Geometry: final body of the model. Coordinates: model frame, mm. Face numbers are marked on the shaded views. A direction names the side the tool comes from. Give positions to 0.01 mm unless a question says otherwise; leave off trailing zeros. Write each loop counter-clockwise with the first axis right and the second up, starting at its lowest first coordinate (ties: lowest second). Pieces come first, ordered by that corner, then holes.
Q1. Cut plane B-B on x = 18.5. Return the cut outline in (y, z).
Q2. Cut plane D-D on x = 40. Return the cut outline in (y, z), plus the area to 3 significant figures.
Q3. Line query: L1, parallel to Y at x = 27, z = 12.5; L2, parallel to Z at x = 16, y = 11; L3, parallel to X at y = 2.5, z = 21.5. Output: solid intervals per line, ascending.
Q4. Reachability of the marked faces 4, 5 and 6 from +Z, -Z, +X, -X, +Y, -Y: full face, straight path, thin tool, end or side. Return the list, or none.
Q5. Draft query along X for the marked faces 1, 2 and 3. Return one class per face: pulls with the +X half, pulls with the -X half, needs draft (parallel to the pull), parting line crosses it, or undercut.
Q6. Cut plane A-A on z = 10.5. Return the cut outline in (x, y), plus the area to 3 significant figures.
Q7. Pin query (flat end, axial travel): pin 1 (5 mm diameter, centred on y = 5, z = 16, fed in from -X); pin 2 (1.5 mm diameter, centred on x = 18, z = 11, fed in from -Y); pin 3 (16 mm diameter, centred on x = 15, z = 11.5, fed in from +Y); pin 4 (6 mm diameter, centred on y = 13, z = 7.5, fed in from +X). Return the tip coordinate at first contact, or that it passes through.
```python
from build123d import *

# Parameters (mm, degrees)
F1_DEPTH  = 32
F2_R      = 16
F3_R      = 15.99999
F4_R      = 16
F5_R      = 15.99999
F6_R      = 8
F7_DEPTH  = 25.4
F8_R      = 8
F9_DEPTH  = 25.4
F10_R     = 12.5095984865
F11_DEPTH = 25.4


# Not quite as in the source:
# - a fillet or chamfer is up to 0.001 mm smaller than in the source, because OpenCascade refuses the exact size


with BuildPart() as f1:
    # F0 (on Top) → F1 (new body)
    with BuildSketch(Plane.XY):
        Polygon((55, -31.1075148418), (55, 19.9773363869), (0, 19.9773363869), (0, 8.9773363869), (44, 8.9773363869), (44, -20.1075148418), (0, -20.1075148418), (0, -31.1075148418), align=None)
    extrude(amount=F1_DEPTH)

    # F2
    f2_edges = [f1.edges().sort_by_distance(p)[0] for p in [
        (0, -25.607515, 32),
    ]]
    fillet(f2_edges, radius=F2_R)

    # F3 (radius 16 in the source; OpenCascade refuses exactly that, so slightly less here)
    f3_edges = [f1.edges().sort_by_distance(p)[0] for p in [
        (0, -25.607515, 0),
    ]]
    fillet(f3_edges, radius=F3_R)

    # F4
    f4_edges = [f1.edges().sort_by_distance(p)[0] for p in [
        (0, 14.477336, 32),
    ]]
    fillet(f4_edges, radius=F4_R)

    # F5 (radius 16 in the source; OpenCascade refuses exactly that, so slightly less here)
    f5_edges = [f1.edges().sort_by_distance(p)[0] for p in [
        (0, 14.477336, 0),
    ]]
    fillet(f5_edges, radius=F5_R)

    # F6 (on face) → F7 (cut)
    with BuildSketch(Plane(origin=(0, 19.9773363869, 0), x_dir=(-1, 0, 0), z_dir=(0, 1, 0))):
        with Locations((-16, 16)):
            Circle(F6_R)
    extrude(amount=-F7_DEPTH, mode=Mode.SUBTRACT)

    # F8 (on face) → F9 (cut)
    with BuildSketch(Plane.XZ.offset(31.1075148418)):
        with Locations((16, 16)):
            Circle(F8_R)
    extrude(amount=-F9_DEPTH, mode=Mode.SUBTRACT)

    # F10 (on face) → F11 (join)
    with BuildSketch(Plane.YZ.offset(55)):
        with Locations((-6.0587972403, 14.9832107127)):
            Circle(F10_R)
    extrude(amount=F11_DEPTH)


solid = f1.part
```
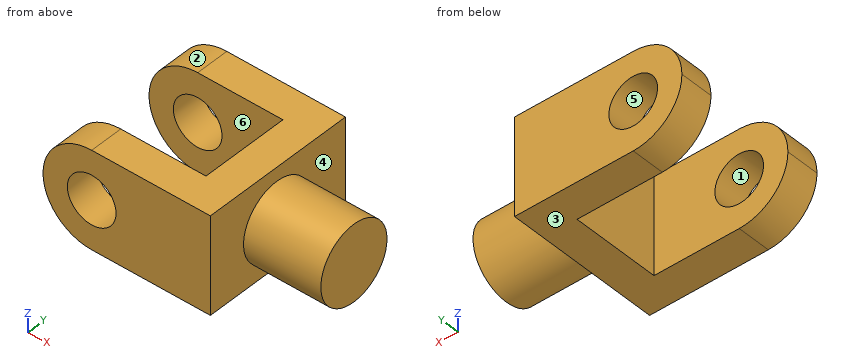
Data:
1. outline: (-31.11, 0) - (-20.11, 0) - (-20.11, 8.4) - (-31.11, 8.4) - close; (-31.11, 23.6) - (-20.11, 23.6) - (-20.11, 32) - (-31.11, 32) - close; (8.98, 0) - (19.98, 0) - (19.98, 8.4) - (8.98, 8.4) - close; (8.98, 23.6) - (19.98, 23.6) - (19.98, 32) - (8.98, 32) - close
2. outline: (-31.11, 0) - (-20.11, 0) - (-20.11, 32) - (-31.11, 32) - close; (8.98, 0) - (19.98, 0) - (19.98, 32) - (8.98, 32) - close
2. area: 704 mm2
3. L1: y = -31.11 to -20.11, 8.98 to 19.98
3. L2: z = 0 to 8, 24 to 32
3. L3: x = 44 to 80.4
4. face 4: +X
4. face 5: +Y, -Y
4. face 6: +Z, -Z, -X
5. face 1: undercut
5. face 2: pulls with the -X half
5. face 3: needs draft
6. outline: (0.98, -31.11) - (10.19, -31.11) - (10.19, -20.11) - (0.98, -20.11) - close; (0.98, 8.98) - (10.19, 8.98) - (10.19, 19.98) - (0.98, 19.98) - close; (21.81, -31.11) - (55, -31.11) - (55, -17.74) - (80.4, -17.74) - (80.4, 5.62) - (55, 5.62) - (55, 19.98) - (21.81, 19.98) - (21.81, 8.98) - (44, 8.98) - (44, -20.11) - (21.81, -20.11) - close
6. area: 1,850 mm2
7. pin 1: stops at x = 44
7. pin 2: passes through
7. pin 3: stops at y = 19.98
7. pin 4: stops at x = 55
